Geometry: final body of the model. Coordinates: model frame, mm. Face numbers are marked on the shaded views. A direction names the side the tool comes from. Give positions to 0.01 mm unless a question says otherwise; leave off trailing zeros. Write each loop counter-clockwise with the first axis right and the second up, starting at its lowest first coordinate (ties: lowest second). Pieces come first, ordered by that corner, then holes. Notation, with made-up numbers: (89.25, 68.25) -> (130.25, 68.25) arc R28 cw to (130.25, 88.25) -> close; hole circle Ø9 at (-10.75, 78.5). An arc over 180 degrees is marked (long way). Answer as a JSON object with one key per item and string values.
Autodesk Inventor part; units mm, degrees
ref_plane "Work Plane1" through (0, 0, 60) normal (-1, 0, 0) x (0, 0, 1)
ref_plane "Work Plane2" through (125, 0, 0) normal (0, 0, -1) x (-1, 0, 0)
ref_plane "Work Plane3" through (-125, 0, 9) normal (0, 0, -1) x (-1, 0, 0)
sketch "Sketch2" plane through (0, 0, 0) normal (0, 1, 0) x (-1, 0, 0)
  line L0 (125, -60) -> (-125, -60)
  line L1 (-125, -60) -> (-125, 60)
  line L2 (-125, 60) -> (125, 60)
  line L3 (125, 60) -> (125, -60)
  point P0 (0, 0)
  point P1 (-125, 0)
  point P2 (0, -60)
  dimension "d2" = 250
  dimension "d3" = 120
extrude "Extrusion1" add sketch "Sketch2" along normal blind 18
sketch "Sketch3" plane through (0, 18, 0) normal (0, 1, 0) x (1, 0, 0)
  line L0 (-125, 60) -> (-41.6667, 60)
  line L1 (-41.6667, 60) -> (-41.6667, 42)
  line L2 (-41.6667, 42) -> (-125, 42)
  line L3 (-125, 42) -> (-125, 60)
  line L4 (125, 60) -> (-125, 60)
  line L5 (-125, 60) -> (-125, -60)
  line L6 (-125, -60) -> (125, -60)
  line L7 (125, -60) -> (125, 60)
  point P0 (0, 0)
  point P1 (-125, 51)
  point P2 (-125, 0)
  point P3 (-83.3333, 60)
  point P4 (0, 60)
  dimension "d6" = 83.3333
  dimension "d7" = 18
extrude "Extrusion2" cut sketch "Sketch3" against normal blind 18 contours L0 L1 L2 L3
ref_plane "Work Plane1" through (0, 0, 60) normal (-1, 0, 0) x (0, 0, 1)
ref_plane "Work Plane2" through (125, 0, 0) normal (0, 0, -1) x (-1, 0, 0)
mirror "Mirror1" about plane through (0, 0, 60) normal (-1, 0, 0) of "Extrusion2"
sketch "Sketch4" plane through (0, 18, 0) normal (0, 1, 0) x (1, 0, 0)
  line L0 (-41.6667, 60) -> (41.6667, 60)
  line L1 (41.6667, 60) -> (41.6667, 51)
  line L2 (41.6667, 51) -> (-41.6667, 51)
  line L3 (-41.6667, 51) -> (-41.6667, 60)
  line L4 (41.6667, 42) -> (41.6667, 60)
  line L5 (41.6667, 60) -> (-41.6667, 60)
  line L6 (-41.6667, 60) -> (-41.6667, 42)
  line L7 (-41.6667, 42) -> (-125, 42)
  line L8 (-125, 42) -> (-125, -60)
  line L9 (-125, -60) -> (125, -60)
  line L10 (125, -60) -> (125, 42)
  line L11 (125, 42) -> (41.6667, 42)
  line L12 (-41.6667, 60) -> (-41.6667, 42)
  point P0 (0, 0)
  point P1 (0, 60)
  point P2 (0, 60)
  point P3 (0, 51)
  point P4 (-41.6667, 51)
  point P5 (41.6667, 55.5)
  point P6 (41.6667, 51)
  point P7 (-41.6667, 55.5)
  point P8 (-41.6667, 51)
extrude "Extrusion3" cut sketch "Sketch4" against normal blind 18 contours L0 L1 L2 L3
sketch "Sketch5" plane through (0, 18, 0) normal (0, 1, 0) x (1, 0, 0)
  line L0 (-41.6667, -60) -> (41.6667, -60)
  line L1 (41.6667, -60) -> (41.6667, -69)
  line L2 (41.6667, -69) -> (-41.6667, -69)
  line L3 (-41.6667, -69) -> (-41.6667, -60)
  line L4 (41.6667, 51) -> (-41.6667, 51)
  line L5 (-41.6667, 51) -> (-41.6667, 42)
  line L6 (-41.6667, 42) -> (-125, 42)
  line L7 (-125, 42) -> (-125, -60)
  line L8 (-125, -60) -> (125, -60)
  line L9 (125, -60) -> (125, 42)
  line L10 (125, 42) -> (41.6667, 42)
  line L11 (41.6667, 42) -> (41.6667, 51)
  line L12 (-125, -60) -> (125, -60)
  point P0 (0, 0)
  point P1 (0, -60)
  point P2 (0, -60)
  point P3 (0, -69)
  point P4 (0, -60)
  dimension "d12" = 83.3333
  dimension "d13" = 9
extrude "Extrusion4" add sketch "Sketch5" against normal blind 18 contours L0 L1 L2 L3
sketch "Sketch6" plane through (0, 18, 0) normal (0, 1, 0) x (1, 0, 0)
  line L0 (-41.6667, 51) -> (-41.6667, 42)
  line L1 (41.6667, 51) -> (41.6667, 42)
  point P0 (0, 0)
  point P1 (-44.8417, 42)
  point P2 (44.8417, 42)
  dimension "d16" = 3.175
  dimension "d17" = 3.175
hole "Hole1" at (-44.8417, 18, -42) at (44.8417, 18, -42) direction (0, -1, 0) diameter 6.35 end through all
ref_plane "Work Plane3" through (-125, 0, 9) normal (0, 0, -1) x (-1, 0, 0)
mirror "Mirror2" about plane through (-125, 0, 9) normal (0, 0, -1) of "Hole1"
equation "\"d2\" = shelfWidth"
equation "\"d3\" = shelfHeight"
equation "\"d4\" = plyThickness"
equation "\"d6\" = 0.333333 * shelfWidth"
equation "\"d7\" = plyThickness"
equation "\"d8\" = plyThickness"
equation "\"d10\" = plyThickness"
equation "\"d12\" = 0.333333 * shelfWidth"
equation "\"d13\" = 0.5 * plyThickness"
equation "\"d14\" = plyThickness"
equation "\"d18\" = millDiameter"
equation "\"plyThickness\" = 18"
equation "\"legHeight\" = 702"
equation "\"millDiameter\" = 6.35"
equation "\"legTopTabHeight\" = 18"
equation "\"legTopSlotDepth\" = 49"
equation "\"shelfWidth\" = 250"
equation "\"shelfHeight\" = 120"
properties part number "shelfSide"
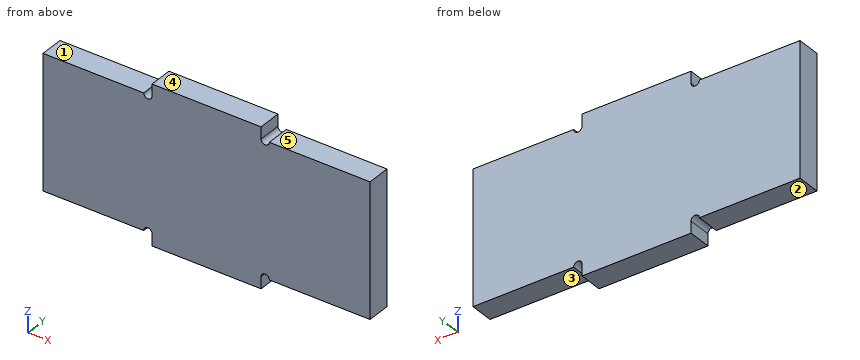
Q1. Cut plane A-A (y = 8). Return the cut outline in (x, z) (3 decimals), and give its area (3 significant figures).
Values:
{"outline": "(-125, -42) -> (-48.017, -42) arc R3.175 cw to (-41.667, -42) -> (-41.667, -51) -> (41.667, -51) -> (41.667, -42) arc R3.175 cw to (48.017, -42) -> (125, -42) -> (125, 60) -> (48.017, 60) arc R3.175 cw to (41.667, 60) -> (41.667, 69) -> (-41.667, 69) -> (-41.667, 60) arc R3.175 cw to (-48.017, 60) -> (-125, 60) -> close", "area": "26,900 mm²"}
Q2. Material intervals for L1, parallel to X at y = 4.25, z = -39.5; L2, parallel to Z at x = -110.5, y = 14.75, sorted ascending. Write a range as from..to.
Values:
{"L1": "-125..-46.8, -42.88..42.88, 46.8..125", "L2": "-42..60"}
Q3. Set-up query: the marked faces 1, 2, 3, 4 and 5. Return all of +Z, -Z, +X, -X, +Y, -Y with unobstructed straight access to the full face (end or side cutting, diameter ignored); none if empty.
Values:
{"face 1": "+Z, -X, +Y, -Y", "face 2": "-Z, -X, +Y, -Y", "face 3": "-Z, +X, +Y, -Y", "face 4": "+Z, +X, -X, +Y, -Y", "face 5": "+Z, +X, +Y, -Y"}
Q4. Cut plane B-B (x = 60.5). Return the cut outline in (y, z), and give its area (3 significant figures).
Values:
{"outline": "(0, -42) -> (18, -42) -> (18, 60) -> (0, 60) -> close", "area": "1,840 mm²"}
Q5. First-contact query: P1, Ø2.5, axis at y = 6.5, z = 64, coming from the +X side; P2, Ø9, axis at x = 76, y = 11.5, coming from the +Z side; P3, Ø9, axis at x = -102, y = 7.5, coming from the -Z side; P4, Ø12, axis at x = -17, z = 54, coming from the -Y side. Flat tips, straight axial feed; report the tip coordinate or a pass-through.
Values:
{"P1": "x = 41.67", "P2": "z = 60", "P3": "z = -42", "P4": "y = 0"}
